Build history of the part. All positions in model axes, mm. Face numbers are marked on the shaded views. A direction names the side the tool comes from. Round coordinates to 2 decimals unless told otherwise and drop trailing zeros. Loops run counter-clockwise (first coordinate to the right, second up) from the corner with the lowest first, then second, coordinate; pieces in that order, holes last. Notation, with made-up numbers: (-0.75, -28) - (19.25, -28) arc R27 cw to (19.25, 10) - close; hole circle Ø3 at (71, 63.5). An arc over 180 degrees is marked (long way). Use a Markdown table: item, result.
from build123d import *

# Parameters (mm, degrees)
BOSS_EXTRUDE1_DEPTH = 1
SKETCH3_R           = 4
BOSS_EXTRUDE2_DEPTH = 10.2
FILLET1_R           = 0.3
SKETCH4_W           = 0.9
SKETCH4_H           = 3.4
BOSS_EXTRUDE3_DEPTH = 0.3
BOSS_EXTRUDE4_DEPTH = 0.01


with BuildPart() as part:
    # Sketch2 → Boss-Extrude1 (new body)
    with BuildSketch(Plane(origin=(0, 0, 0), x_dir=(1, 0, 0), z_dir=(0, 1, 0))):
        Polygon((4.15, -4.15), (-4.15, -4.15), (-4.15, 3.1), (-3.1, 4.15), (3.1, 4.15), (4.15, 3.1), align=None)
    extrude(amount=BOSS_EXTRUDE1_DEPTH)

    # Sketch3 → Boss-Extrude2 (add)
    with BuildSketch(Plane(origin=(0, 0, 0), x_dir=(1, 0, 0), z_dir=(0, 1, 0))):
        Circle(SKETCH3_R)
    extrude(amount=BOSS_EXTRUDE2_DEPTH)

    # Fillet1
    fillet1_edges = [part.edges().sort_by_distance(p)[0] for p in [
        (-4, 10.2, 0),
    ]]
    fillet(fillet1_edges, radius=FILLET1_R)

    # Sketch4 → Boss-Extrude3 (add)
    with BuildSketch(Plane(origin=(0, 0, 0), x_dir=(1, 0, 0), z_dir=(0, 1, 0))):
        with Locations((0, 3.25)):
            Rectangle(SKETCH4_W, SKETCH4_H)
        with Locations((0, -3.25)):
            Rectangle(SKETCH4_W, SKETCH4_H)
    extrude(amount=BOSS_EXTRUDE3_DEPTH)

    # Sketch5 → Boss-Extrude4 (add)
    with BuildSketch(Plane(origin=(0, 10.2, 0), x_dir=(1, 0, 0), z_dir=(0, 1, 0))):
        with BuildLine():
            Line((-3.190682189, -1.873378544), (3.190682189, -1.873378544))
            ThreePointArc((3.190682189, -1.873378544), (0, -3.7), (-3.190682189, -1.873378544))
        make_face()
    extrude(amount=BOSS_EXTRUDE4_DEPTH)


solid = part.part
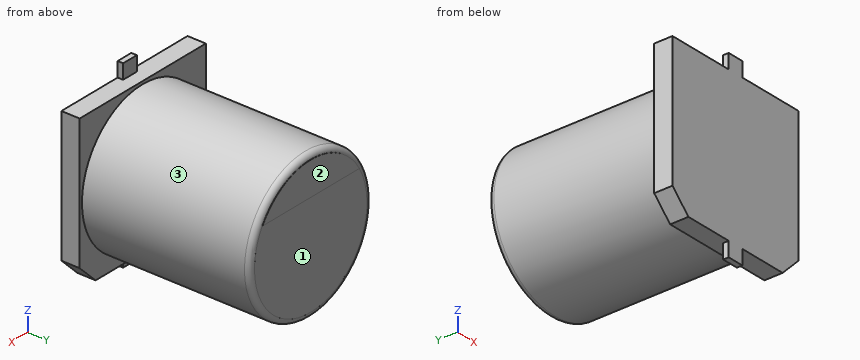
Q1. Cut at B-B, the plane z = 0. List the corners of the cut face in (x, y), plus the area to 3 significant figures.
Results found:
| item | result |
|---|---|
| outline | (-4.15, 0) - (4.15, 0) - (4.15, 1) - (4, 1) - (4, 9.9) arc R0.3 ccw to (3.7, 10.2) - (-3.7, 10.2) arc R0.3 ccw to (-4, 9.9) - (-4, 1) - (-4.15, 1) - close |
| area | 81.9 mm2 |
Q2. Probe line 1 (Y direction, x = -0.75, z = -2); line 2 (Z direction, x = -3, y = 0.5); line 3 (Y direction, x = 3.75, z = -2). List the from-to ranges inside material, lowest first.
Results found:
| item | result |
|---|---|
| line 1 | y = 0 to 10.2 |
| line 2 | z = -4.15 to 4.15 |
| line 3 | y = 0 to 1 |
Q3. Which spindle directions (+Z, -Z, +X, -X, +Y, -Y) get a long thin tool onto all of the face, cutting with end or side? Do the marked faces 1, 2 and 3. Say none if no direction does.
Results found:
| item | result |
|---|---|
| face 1 | -Z, +X, -X, +Y |
| face 2 | +Z, -Z, +X, -X, +Y |
| face 3 | +Y |
Q4. Cut at C-C, the plane y = 6.75. List the corners of the cut face in (x, z).
Results found:
| item | result |
|---|---|
| outline | circle Ø8 at (0, 0) |
Q5. Drop flat-ended pins along their axis: pin 1 (3 mm diameter, centred on x = 0, y = 8, fed in from +Z); pin 2 (2.5 mm diameter, centred on x = 1.5, z = 0.5, fed in from +Y); pin 3 (0.5 mm diameter, centred on x = 0.5, y = 0.5, fed in from -Z); pin 4 (3 mm diameter, centred on x = -1, y = 2, fed in from -Z). Give the stop position or say it passes through.
Results found:
| item | result |
|---|---|
| pin 1 | stops at z = 4 |
| pin 2 | stops at y = 10.2 |
| pin 3 | stops at z = -4.95 |
| pin 4 | stops at z = -4.15 |
